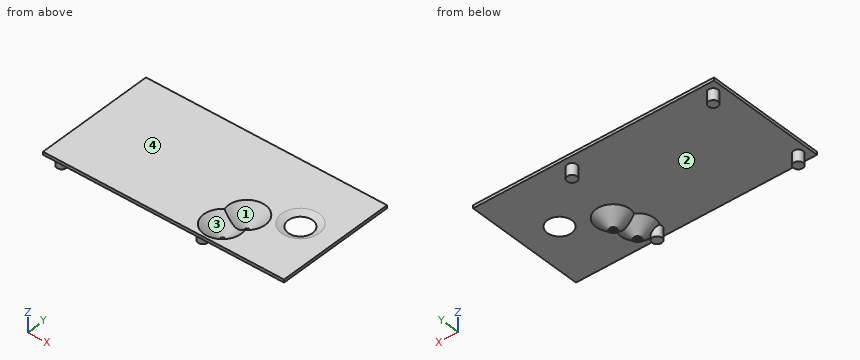
from build123d import *

# Parameters (mm, degrees)
SKETCH001_W                    = 160.5
SKETCH001_H                    = 2
PAD001_DEPTH                   = 40
CYLINDER_R                     = 3.25
CYLINDER_DEPTH                 = 7.65
CYLINDER_LINEARPATTERN_2_R     = 3.25
CYLINDER_LINEARPATTERN_2_DEPTH = 7.65


with BuildPart() as part:
    # Sketch001 → Pad001 (new body, symmetric)
    with BuildSketch(Plane.XZ):
        with Locations((-20.25, 21.5)):
            Rectangle(SKETCH001_W, SKETCH001_H)
    extrude(amount=PAD001_DEPTH, both=True)

    # Cone002 → Cone002 (revolve)
    with BuildSketch(Plane(origin=(11.4, -12.2, 12.75), x_dir=(1, 0, 0), z_dir=(0, -1, 0))):
        Polygon((0, 0), (2.5, 0), (12.5, 8.75), (0, 8.75), align=None)
    revolve(axis=Axis((11.4, -12.2, 12.75), (0, 0, 1)))

    # Cone003 → Cone003 (revolve)
    with BuildSketch(Plane(origin=(6.85, -25.85, 12.75), x_dir=(1, 0, 0), z_dir=(0, -1, 0))):
        Polygon((0, 0), (2.5, 0), (12.5, 8.75), (0, 8.75), align=None)
    revolve(axis=Axis((6.85, -25.85, 12.75), (0, 0, 1)))

    # Cylinder → Cylinder (join)
    with BuildSketch(Plane(origin=(0, -33.025, 20.5), x_dir=(1, 0, 0), z_dir=(0, 0, -1))):
        Circle(CYLINDER_R)
    cylinder = extrude(amount=CYLINDER_DEPTH)

    # Cylinder LinearPattern 2 → Cylinder LinearPattern 2 (add)
    with BuildSketch(Plane(origin=(-94, -33.025, 20.5), x_dir=(1, 0, 0), z_dir=(0, 0, -1))):
        Circle(CYLINDER_LINEARPATTERN_2_R)
    cylinder_linearpattern_2 = extrude(amount=CYLINDER_LINEARPATTERN_2_DEPTH)

    # Mirrored: Cylinder, Cylinder LinearPattern 2 across XZ
    add(cylinder.mirror(Plane.XZ))
    add(cylinder_linearpattern_2.mirror(Plane.XZ))

    # Cone001 → Cone001 (revolve, cut)
    with BuildSketch(Plane(origin=(11.4, -12.2, 12.75), x_dir=(1, 0, 0), z_dir=(0, -1, 0))):
        Polygon((0, 0), (1.5, 0), (13.5, 10.75), (0, 10.75), align=None)
    revolve(axis=Axis((11.4, -12.2, 12.75), (0, 0, 1)), mode=Mode.SUBTRACT)

    # Cone004 → Cone004 (revolve, cut)
    with BuildSketch(Plane(origin=(6.85, -25.85, 12.75), x_dir=(1, 0, 0), z_dir=(0, -1, 0))):
        Polygon((0, 0), (1.5, 0), (13.5, 10.75), (0, 10.75), align=None)
    revolve(axis=Axis((6.85, -25.85, 12.75), (0, 0, 1)), mode=Mode.SUBTRACT)

    # Cone → Cone (revolve, cut)
    with BuildSketch(Plane(origin=(36.525, 0.15, 17.5), x_dir=(1, 0, 0), z_dir=(0, -1, 0))):
        Polygon((0, 0), (1.5, 0), (12.5, 5), (0, 5), align=None)
    revolve(axis=Axis((36.525, 0.15, 17.5), (0, 0, 1)), mode=Mode.SUBTRACT)


solid = part.part
The model under review builds one solid part; all positions refer to its coordinate system, in mm. Face numbers are marked on the shaded views. A direction names the side the tool comes from. Round coordinates to 2 decimals unless told otherwise and drop trailing zeros. Loops run counter-clockwise (first coordinate to the right, second up) from the corner with the lowest first, then second, coordinate; pieces in that order, holes last. Notation, with made-up numbers: (-12.75, 65) -> (-1.75, 65) arc R16 cw to (-1.75, 78) -> close; hole circle Ø5 at (81, 84.25). An arc over 180 degrees is marked (long way). Write item = value, one per line. Start each with the question number.
Item 1: Take a section at C-C on x = -60. Give the boundary of the cut face in (y, z).
Item 2: Mouldability with a two-part tool opening along X and no side actions: class the marked faces 3 and 4 as released by +X, released by -X, zero draft, split by the parting line, or undercut.
Item 3: To check wall thickness, follow L1, parallel to Z at x = -42.5, y = 0.5; L2, parallel to X at y = 34.5, z = 16.5; L3, parallel to X at y = -29, z = 15.25. State the ranges of each line that lie inside material, in increasing order.
Item 4: Insertion check: pin 1 (5 mm diameter, centred on x = 0.5, y = 34, fed in from -Z); pin 2 (3 mm diameter, centred on y = -22.5, z = 17, fed in from +X). Each pin has a flat end and moves straight along its axis. Give the tip position at first contact, or say it passes through.
Item 5: For the marked faces 1 and 2, list the 3-axis set-ups (+Z, -Z, +X, -X, +Y, -Y) from which the entire face can be reached by the end or side of a thin tool; tool diameter is ignored.
Item 6: Take a section at A-A on y = -25.85. Give the boundary of the cut face in (x, z), plus the area to 3 significant figures.
Item 7: Take a section at B-B on x = -94. Give the boundary of the cut face in (y, z) (3 decimals).
Result:
q1.outline = (-40, 20.5) -> (40, 20.5) -> (40, 22.5) -> (-40, 22.5) -> close
q2.face_3 = undercut
q2.face_4 = zero draft
q3.L1 = 20.5 to 22.5
q3.L2 = -96.9 to -91.1, -2.9 to 2.9
q3.L3 = 2.52 to 3.94, 9.76 to 11.18
q4.pin_1 = 12.85
q4.pin_2 = 15.36
q5.face_1 = +Z
q5.face_2 = -Z
q6.outline = (-100.5, 20.5) -> (-4.51, 20.5) -> (4.35, 12.75) -> (5.35, 12.75) -> (-5.53, 22.5) -> (-100.5, 22.5) -> close; (8.35, 12.75) -> (9.35, 12.75) -> (18.21, 20.5) -> (60, 20.5) -> (60, 22.5) -> (19.23, 22.5) -> close
q6.area = 293 mm²
q7.outline = (-40, 20.5) -> (-36.275, 20.5) -> (-36.275, 12.85) -> (-29.775, 12.85) -> (-29.775, 20.5) -> (29.775, 20.5) -> (29.775, 12.85) -> (36.275, 12.85) -> (36.275, 20.5) -> (40, 20.5) -> (40, 22.5) -> (-40, 22.5) -> close
